from build123d import *

# Parameters (mm, degrees)
F0_W     = 400
F0_H     = 600
F1_DEPTH = 80
F2_T     = -5


with BuildPart() as f1:
    # F0 (on Top) → F1 (new body)
    with BuildSketch(Plane.XY):
        Rectangle(F0_W, F0_H)
    extrude(amount=F1_DEPTH)

    # F2
    f2_openings = [f1.faces().sort_by_distance(p)[0] for p in [
        (0, 0, 80),
    ]]
    offset(amount=F2_T, openings=f2_openings)


with BuildPart() as f3_1:
    # F3: copy of F1
    add(f1.part.moved(Location((0, 0, 90))))


solid = f1.part
Model file for the job. Use its own axes, mm. A direction names the side the tool comes from. Give positions to 0.01 mm unless a question says otherwise; leave off trailing zeros. Order: outer loops, then holes, each group sorted by start corner. A loop starts at its lowest first (then second) coordinate and runs counter-clockwise, first axis right, second up. Notation, with made-up numbers: (-33, -37.75) - (12, -37.75) arc R20 cw to (12, -2.75) - close; hole circle Ø6 at (17.25, 42.25). An arc over 180 degrees is marked (long way). One line per item, written item: value.
Item 1: Tool access for faces 1 (the flat face through (-3, -295, 42)), 2 (the flat face through (-3, 300, 39)): list every direction of +Z, -Z, +X, -X, +Y, -Y with a clear straight run to the whole face (end or side of a thin tool).
Response values:
face 1: +Z
face 2: +Z, -Z, +X, -X, +Y
Item 2: Pin check, flat tip, straight feed: pin 1 Ø10 at (x, y) = (-78.5, -176) entering from +Z. Stop position of the tip, or through.
Response values:
pin 1: z = 5
Item 3: Two-plate mould, pull along X, no slides. Class faces 3 (the flat face through (-3, -300, 39)), 4 (the flat face through (195, -4, 42)), 5 (the flat face through (-200, -4, 39)): released by +X, released by -X, zero draft, split by the parting line, or undercut.
Response values:
face 3: zero draft
face 4: undercut
face 5: released by -X
Item 4: Slice it at A-A (z = 31.5). List the corners of the cut face in (x, y).
Response values:
outline: (-200, -300) - (200, -300) - (200, 300) - (-200, 300) - close; hole (-195, -295) - (195, -295) - (195, 295) - (-195, 295) - close
Item 5: Slice it at C-C (x = -141). List the corners of the cut face in (y, z).
Response values:
outline: (-300, 0) - (300, 0) - (300, 80) - (295, 80) - (295, 5) - (-295, 5) - (-295, 80) - (-300, 80) - close
Item 6: Wall check: line 1 (X direction, y = -115.5, z = 27); line 2 (Y direction, x = 173, z = 32); line 3 (Z direction, x = 19, y = -34.5). Give the ranges that are in metal, low to high.
Response values:
line 1: -200 to -195, 195 to 200
line 2: -300 to -295, 295 to 300
line 3: 0 to 5
Item 7: Slice it at B-B (y = -229.5). List the corners of the cut face in (x, z), then the cut area to 3 significant figures.
Response values:
outline: (-200, 0) - (200, 0) - (200, 80) - (195, 80) - (195, 5) - (-195, 5) - (-195, 80) - (-200, 80) - close
area: 2,750 mm2
